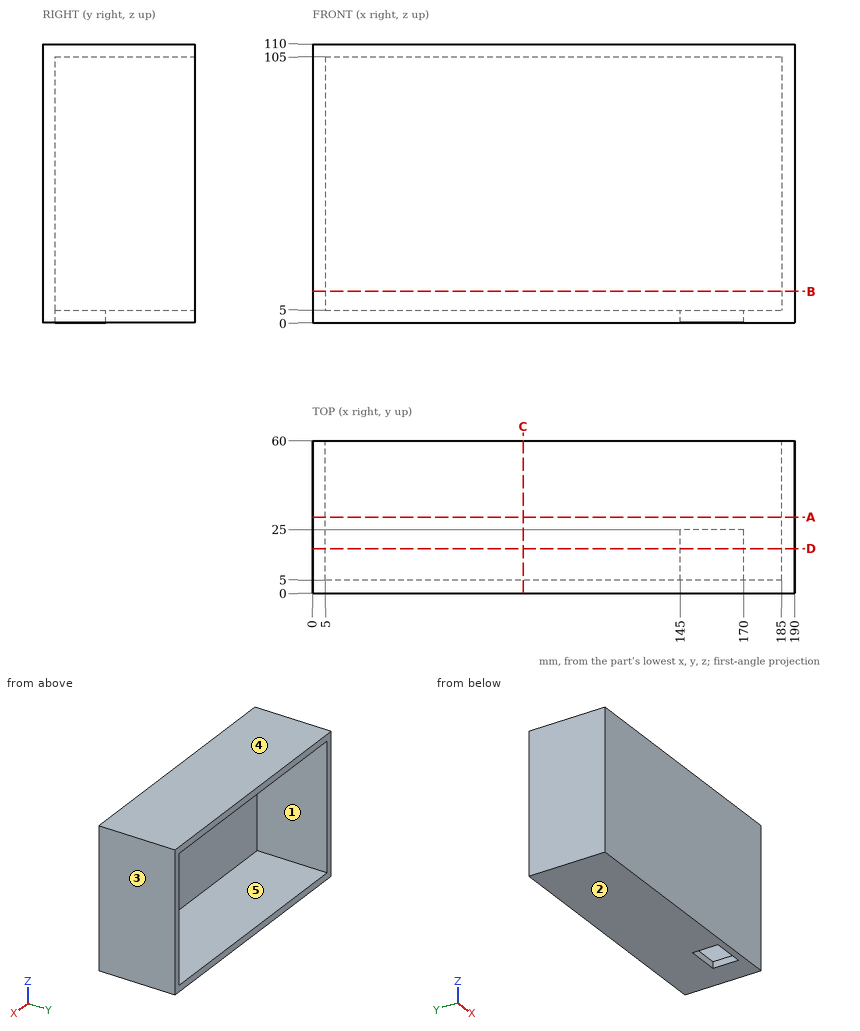
Print and shaded views of the part. All mm, measured from the part's lowest x, y and z. A direction names the side the tool comes from. Coordinates: 2 decimals unless noted, no trailing zeros. Order: outer loops, then holes, each group sorted by start corner. A loop starts at its lowest first (then second) coordinate and runs counter-clockwise, first axis right, second up. Notation, with made-up numbers: M -26.75,47 L -9.75,47 A20 cw -9.75,74 Z; hole C 44.5,-27 d1. An arc over 180 degrees is marked long. One line per question, with ' | ' between items. Start each with the question number.
Q1. 3-axis set-ups, long thin cutter, end or side, ignore diameter. For the marked faces 1 and 2: which of +Z, -Z, +X, -X, +Y, -Y reach the whole face in a straight line?
Q2. Probe L1, parallel to X at y = 39, z = 75.5; L2, parallel to Z at x = 18.5, y = 54.5; L3, parallel to Y at x = 18.5, z = 69. List the from-to ranges inside material, lowest first. Write a range as from..to.
Q3. Saw through at C-C (x = 83). List the corners of the cut face in (y, z), then the cut area to 3 significant figures.
Q4. Flat gauge pins, fed straight in: pin 1 Ø2.5 at (x, z) = (159, 2) entering from -Y; pin 2 Ø5 at (x, z) = (20.5, 13) entering from +Y. Where does each tip first touch, or does it go through?
Q5. Two-plate mould, pull along X, no slides. Class the marked faces 3, 4 and 5: +X half, -X half, draft (parallel to the pull), parting line (faces both ways), or undercut.
Q6. Saw through at A-A (y = 30). List the corners of the cut face in (x, z).
Q7. Saw through at D-D (y = 17.5). List the corners of the cut face in (x, z), then the cut area to 4 significant figures.
Q8. Saw through at B-B (z = 12.5). List the corners of the cut face in (x, y).
Check values:
1) face 1: +Y | face 2: -Z, +X, -X, +Y, -Y
2) L1: x = 0..5, 185..190 | L2: z = 0..5, 105..110 | L3: y = 0..5
3) outline: M 0,0 L 60,0 L 60,5 L 5,5 L 5,105 L 60,105 L 60,110 L 0,110 Z | area: 1,100 mm2
4) pin 1: stops at y = 0 | pin 2: stops at y = 5
5) face 3: +X half | face 4: draft | face 5: undercut
6) outline: M 0,0 L 190,0 L 190,110 L 0,110 Z; hole M 5,5 L 185,5 L 185,105 L 5,105 Z
7) outline: M 0,0 L 145,0 L 145,5 L 5,5 L 5,105 L 185,105 L 185,5 L 170,5 L 170,0 L 190,0 L 190,110 L 0,110 Z | area: 2,775 mm2
8) outline: M 0,0 L 190,0 L 190,60 L 185,60 L 185,5 L 5,5 L 5,60 L 0,60 Z
